Work out the finished part from the listing and answer in its coordinate system (mm). A direction names the side the tool comes from. Give positions to 0.01 mm unless a question says otherwise; leave off trailing zeros. Loops run counter-clockwise (first coordinate to the right, second up) from the corner with the lowest first, then second, coordinate; pieces in that order, holes last. Notation, with made-up numbers: (21.5, 2.5) - (33.5, 2.5) arc R25 cw to (33.5, 28.5) - close; hole circle Ø7 at (19, -30.5). An arc over 180 degrees is marked (long way). One line per question, with ' | ' between items.
from build123d import *
from build123d.topology import SkipClean

# Parameters (mm, degrees)
BASPROSKE_W         = 5
BASPROSKE_H         = 5.5
TOOTHCUT_DEPTH      = 10.246621004
TEETHCUTS_COUNT     = 20
TEETHCUTS_ANGLE     = 342
HUBNEAONESKE_R      = 4.374
HUBNEARONE_DEPTH    = 5.0000508
BORSKE_R            = 2.5
BORE_DEPTH          = 10.0000508
SKETCH_1_R          = 5.5
CUT_EXTRUDE_1_DEPTH = 1


with BuildPart() as part:
    # BasProSke → Base-Revolve (revolve)
    with BuildSketch(Plane(origin=(0, 0, 0), x_dir=(1, 0, 0), z_dir=(0, 1, 0)), mode=Mode.PRIVATE) as base_revolve_sk:
        with Locations((2.5, 2.75)):
            Rectangle(BASPROSKE_W, BASPROSKE_H)
    revolve(base_revolve_sk.sketch.rotate(Axis((-10, 0, 0), (1, 0, 0)), 180), axis=Axis((-10, 0, 0), (1, 0, 0)))

    # TooCutSke → ToothCut (cut, through all)
    with BuildSketch(Plane(origin=(0, 0, 0), x_dir=(0, 0, -1), z_dir=(1, 0, 0))):
        with BuildLine():
            ThreePointArc((0.249903181, 4.366855207), (0, 4.374), (-0.249903181, 4.366855207))
            ThreePointArc((-0.249903181, 4.366855207), (-0.415207844, 4.95951031), (-0.752843848, 5.473871692))
            ThreePointArc((-0.752843848, 5.473871692), (0, 5.5254), (0.752843848, 5.473871692))
            ThreePointArc((0.752843848, 5.473871692), (0.415207844, 4.95951031), (0.249903181, 4.366855207))
        make_face()
    toothcut = extrude(amount=TOOTHCUT_DEPTH, mode=Mode.SUBTRACT)

    # TeethCuts: ToothCut ×20 about axis
    teethcuts_axis = Axis((-10, 0, 0), (1, 0, 0))
    for i in range(1, TEETHCUTS_COUNT):
        add(toothcut.rotate(teethcuts_axis, i * TEETHCUTS_ANGLE / (TEETHCUTS_COUNT - 1)), mode=Mode.SUBTRACT)

    # HubNeaOneSke → HubNearOne (add)
    with SkipClean():  # the faces are left unmerged after this step: merging them gives an invalid solid
        with BuildSketch(Plane.ZY):
            Circle(HUBNEAONESKE_R)
        extrude(amount=HUBNEARONE_DEPTH)

    # BorSke → Bore (cut, symmetric)
    with SkipClean():  # the faces are left unmerged after this step: merging them gives an invalid solid
        with BuildSketch(Plane(origin=(0, 0, 0), x_dir=(0, 0, -1), z_dir=(1, 0, 0))):
            with Locations(Location((0, 0, 0), (0, 0, 180))):
                Circle(BORSKE_R)
        extrude(amount=BORE_DEPTH, both=True, mode=Mode.SUBTRACT)

    # 草图1 → 切除-拉伸1 (cut)
    with SkipClean():  # the faces are left unmerged after this step: merging them gives an invalid solid
        with BuildSketch(Plane(origin=(5, 0, 0), x_dir=(0, 0, -1), z_dir=(1, 0, 0))):
            Circle(SKETCH_1_R)
        extrude(amount=-CUT_EXTRUDE_1_DEPTH, mode=Mode.SUBTRACT)


solid = part.part
1. Find section C-C on x = -0.75. Write down the section's boundary in (y, z).
Evaluation:
outline: circle Ø8.75 at (0, 0); hole circle Ø5 at (0, 0)
2. Find section A-A on y = 0. Write down the section's boundary in (x, z), then the cut area to 3 significant figures.
Evaluation:
outline: (-5, -4.37) - (4, -4.37) - (4, -2.5) - (-5, -2.5) - close; (-5, 2.5) - (4, 2.5) - (4, 4.37) - (-5, 4.37) - close | area: 33.7 mm2
3. Determine the mould class of faces 1 (the cylindrical face through (1.972, 0.406, -4.938)), 2 (the cylindrical face through (1.972, -0.406, 4.938)), 3 (the cylindrical face through (1.972, 4.233, -2.574)), 4 (the flat face through (0, -0.8, 4.8)) for opening direction Z: +Z half, -Z half, draft (parallel to the pull), parting line (faces both ways), or undercut.
Evaluation:
face 1: -Z half | face 2: +Z half | face 3: undercut | face 4: draft
4. Consider L1, parallel to Y at x = -2, z = 0; L2, parallel to Y at x = -3.5, z = -3.5. Determine where each line is inside the solid, lowest interval first.
Evaluation:
L1: -4.37 to -2.5, 2.5 to 4.37 | L2: -2.62 to 2.62
5. Which of the six approach directions +Z, -Z, +X, -X, +Y, -Y give full straight-line access (tool end or side, diameter ignored) to faces 5 (the cylindrical face through (1.972, 4.938, 0.406)), 6 (the flat face through (0, 2.2, -4.3)), 7 (the cylindrical face through (1.97, -4.57, -1.91)), 8 (the cylindrical face through (1.972, -2.574, -4.233))?
Evaluation:
face 5: +X, -X, +Y | face 6: -Z, -X, +Y | face 7: +X, -X, -Y | face 8: +X, -X
6. Flat-ended cylindrical pins translate along their axes: pin 1 (1 mm diameter, centred on y = -0.5, z = 5, fed in from -X); pin 2 (1 mm diameter, centred on x = -3.5, y = 0.5, fed in from +Z); pin 3 (2 mm diameter, centred on x = 0.5, z = -4, fed in from -Y). Find the tip coordinate at first contact, or state that the pin passes through.
Evaluation:
pin 1: x = 0 | pin 2: z = 4.37 | pin 3: y = -3.98
7. Find section D-D on y = 1.75. Write down the section's boundary in (x, z), then the cut area to 3 significant figures.
Evaluation:
outline: (-5, -4.01) - (0, -4.01) - (0, -4.36) - (4, -4.36) - (4, -1.79) - (-5, -1.79) - close; (-5, 1.79) - (4, 1.79) - (4, 4.36) - (0, 4.36) - (0, 4.01) - (-5, 4.01) - close | area: 42.9 mm2
